Job drawing, mm, ordinate dimensions from the low corner. One solid piece. Round coordinates to 2 decimals unless told otherwise and drop trailing zeros. Loops run counter-clockwise (first coordinate to the right, second up) from the corner with the lowest first, then second, coordinate; pieces in that order, holes last.
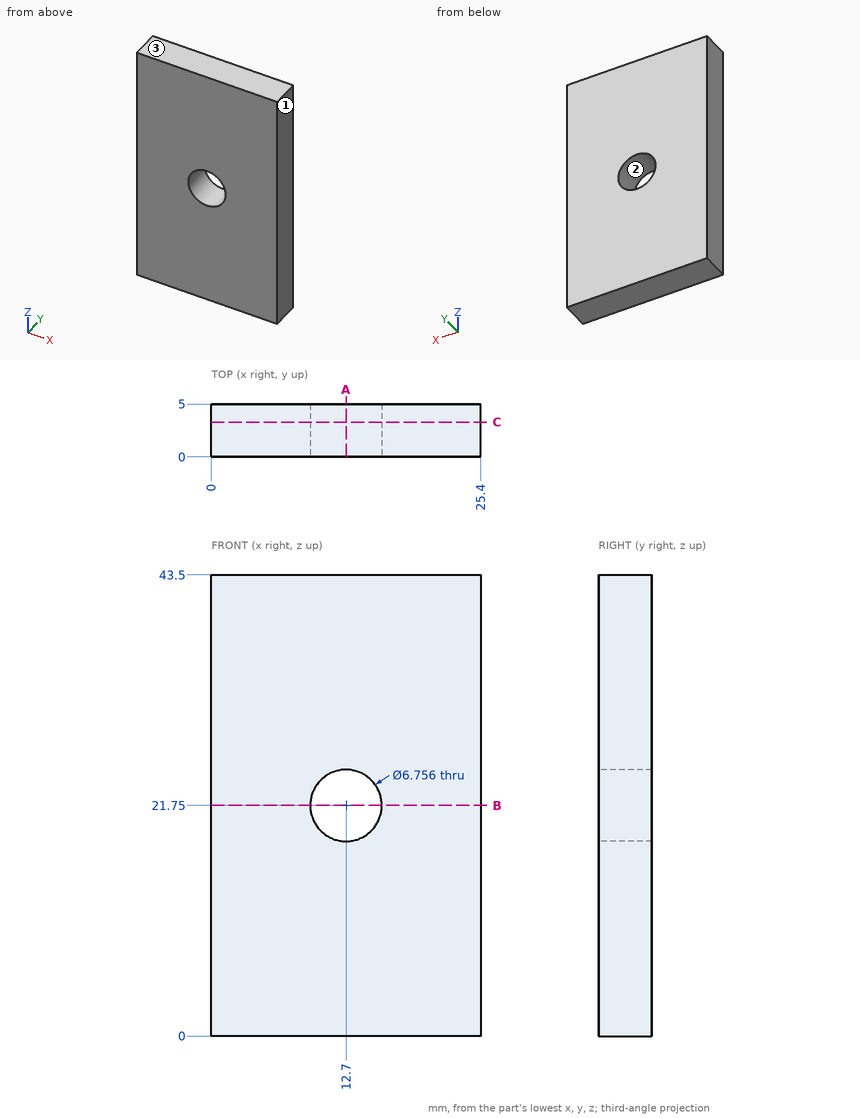
(1) Slice it at C-C on y = 3.3. List the corners of the cut face in (x, z), plus the area to 3 significant figures.
Responses:
outline: (0, 0) - (25.4, 0) - (25.4, 43.5) - (0, 43.5) - close; hole circle Ø6.76 at (12.7, 21.75)
area: 1,070 mm2
(2) Slice it at A-A on x = 12.7. List the corners of the cut face in (y, z), plus the area to 3 significant figures.
Responses:
outline: (0, 0) - (5, 0) - (5, 18.37) - (0, 18.37) - close; (0, 25.13) - (5, 25.13) - (5, 43.5) - (0, 43.5) - close
area: 184 mm2
(3) Probe line 1 (X direction, y = 1.55, z = 21.75); line 2 (Z direction, x = 12.7, y = 3.5); line 3 (Z direction, x = 13.75, y = 3.25). List the from-to ranges inside material, lowest first.
Responses:
line 1: x = 0 to 9.32, 16.08 to 25.4
line 2: z = 0 to 18.37, 25.13 to 43.5
line 3: z = 0 to 18.54, 24.96 to 43.5
(4) Slice it at B-B on z = 21.75. List the corners of the cut face in (x, y).
Responses:
outline: (0, 0) - (9.32, 0) - (9.32, 5) - (0, 5) - close; (16.08, 0) - (25.4, 0) - (25.4, 5) - (16.08, 5) - close
(5) Pull direction Z, two halves, no side cores. Call the marked faces 1, 2 and 3: +Z half, -Z half, draft (parallel to the pull), parting line (faces both ways), or undercut.
Responses:
face 1: draft
face 2: undercut
face 3: +Z half
